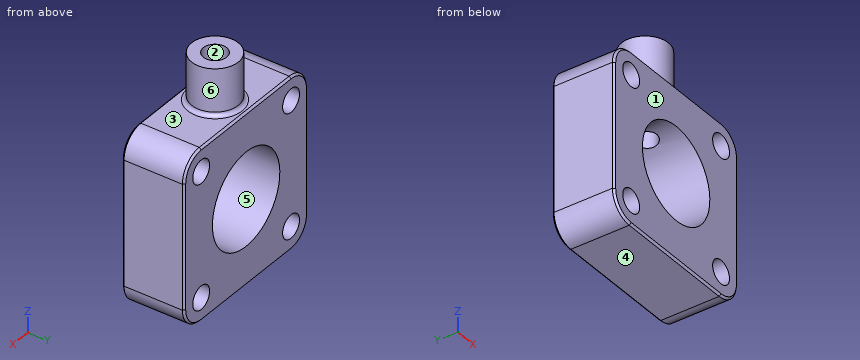
```python
from build123d import *

# Parameters (mm, degrees)
SKETCH1_R           = 1.5
SKETCH1_R_2         = 6
BOSS_EXTRUDE1_DEPTH = 4
BOSS_EXTRUDE2_START = 11
SKETCH2_R           = 3
BOSS_EXTRUDE2_DEPTH = 6
SKETCH3_R           = 1.5
CUT_EXTRUDE1_DEPTH  = 16
CHAMFER1_SIZE       = 0.25
FILLET1_R           = 0.5


with BuildPart() as part:
    # Sketch1 → Boss-Extrude1 (new, symmetric)
    with BuildSketch(Plane(origin=(0, 0, 0), x_dir=(1, 0, 0), z_dir=(0, 1, 0))):
        with BuildLine():
            Line((8, -11), (-8, -11))
            ThreePointArc((-8, -11), (-10.121320344, -10.121320344), (-11, -8))
            Line((-11, -8), (-11, 8))
            ThreePointArc((-11, 8), (-10.121320344, 10.121320344), (-8, 11))
            Line((-8, 11), (8, 11))
            ThreePointArc((8, 11), (10.121320344, 10.121320344), (11, 8))
            Line((11, 8), (11, -8))
            ThreePointArc((11, -8), (10.121320344, -10.121320344), (8, -11))
        make_face()
        with Locations(Location((-8, 8, 0), (0, 0, 270))):
            Circle(SKETCH1_R, mode=Mode.SUBTRACT)
        with Locations(Location((8, 8, 0), (0, 0, 270))):
            Circle(SKETCH1_R, mode=Mode.SUBTRACT)
        with Locations(Location((8, -8, 0), (0, 0, 270))):
            Circle(SKETCH1_R, mode=Mode.SUBTRACT)
        with Locations(Location((-8, -8, 0), (0, 0, 270))):
            Circle(SKETCH1_R, mode=Mode.SUBTRACT)
        with Locations(Location((0, 0, 0), (0, 0, 270))):
            Circle(SKETCH1_R_2, mode=Mode.SUBTRACT)
    extrude(amount=BOSS_EXTRUDE1_DEPTH, both=True)

    # Sketch2 → Boss-Extrude2 (add)
    with BuildSketch(Plane.XY.offset(BOSS_EXTRUDE2_START)):
        with Locations(Location((0, 0, 0), (0, 0, 180))):
            Circle(SKETCH2_R)
    extrude(amount=BOSS_EXTRUDE2_DEPTH)

    # Sketch3 → Cut-Extrude1 (cut)
    with BuildSketch(Plane.XY.offset(17)):
        Circle(SKETCH3_R)
    extrude(amount=-CUT_EXTRUDE1_DEPTH, mode=Mode.SUBTRACT)

    # Chamfer1
    chamfer1_edges = [part.edges().sort_by_distance(p)[0] for p in [
        (0, -4, -11),
        (10.121320344, -4, -10.121320344),
        (11, -4, 0),
        (10.121320344, -4, 10.121320344),
        (10.121320344, 4, -10.121320344),
        (0, 4, -11),
        (-10.121320344, 4, -10.121320344),
        (-11, 4, 0),
        (-10.121320344, 4, 10.121320344),
        (0, 4, 11),
        (10.121320344, 4, 10.121320344),
        (0, -4, 11),
        (11, 4, 0),
        (-10.121320344, -4, 10.121320344),
        (-11, -4, 0),
        (-10.121320344, -4, -10.121320344),
    ]]
    chamfer(chamfer1_edges, length=CHAMFER1_SIZE)

    # Fillet1
    fillet1_edges = [part.edges().sort_by_distance(p)[0] for p in [
        (3, 0, 11),
    ]]
    fillet(fillet1_edges, radius=FILLET1_R)


solid = part.part
```
Verification items for the finished model (mm, model axes). Face numbers are marked on the shaded views. A direction names the side the tool comes from. Round coordinates to 2 decimals unless told otherwise and drop trailing zeros. Order: outer loops, then holes, each group sorted by start corner. A loop starts at its lowest first (then second) coordinate and runs counter-clockwise, first axis right, second up.
1) Depth check by flat-ended pin: pin 1 (2.5 mm diameter, centred on x = 0, y = 0, fed in from +Z). Enter the tip coordinate at first touch or a pass-through.
Geometry says:
pin 1: stops at z = -5.87
2) Cross-section at A-A, the plane x = 0. Record the cut outline in (y, z).
Geometry says:
outline: (-4, -10.75) - (-3.75, -11) - (3.75, -11) - (4, -10.75) - (4, -6) - (-4, -6) - close; (-4, 6) - (-1.5, 6) - (-1.5, 17) - (-3, 17) - (-3, 11.5) arc R0.5 cw to (-3.5, 11) - (-3.75, 11) - (-4, 10.75) - close; (1.5, 6) - (4, 6) - (4, 10.75) - (3.75, 11) - (3.5, 11) arc R0.5 cw to (3, 11.5) - (3, 17) - (1.5, 17) - close
3) Draft check along Z on the marked faces 3, 4, 5 and 6. Enter one of: +Z half, -Z half, draft (parallel to the pull), parting line (faces both ways), or undercut.
Geometry says:
face 3: +Z half
face 4: -Z half
face 5: undercut
face 6: draft
4) Cross-section at C-C, the plane x = -4. Record the cut outline in (y, z), plus the area to 3 significant figures.
Geometry says:
outline: (-4, -10.75) - (-3.75, -11) - (3.75, -11) - (4, -10.75) - (4, -4.47) - (-4, -4.47) - close; (-4, 4.47) - (4, 4.47) - (4, 10.75) - (3.75, 11) - (-3.75, 11) - (-4, 10.75) - close
area: 104 mm2
5) Cross-section at B-B, the plane y = 0. Record the cut outline in (x, z).
Geometry says:
outline: (-11, -8) arc R3 ccw to (-8, -11) - (8, -11) arc R3 ccw to (11, -8) - (11, 8) arc R3 ccw to (8, 11) - (3.5, 11) arc R0.5 cw to (3, 11.5) - (3, 17) - (1.5, 17) - (1.5, 5.81) arc R6 cw (long way) to (-1.5, 5.81) - (-1.5, 17) - (-3, 17) - (-3, 11.5) arc R0.5 cw to (-3.5, 11) - (-8, 11) arc R3 ccw to (-11, 8) - close; hole circle Ø3 at (-8, -8); hole circle Ø3 at (-8, 8); hole circle Ø3 at (8, -8); hole circle Ø3 at (8, 8)
6) Tool access check on the marked faces 1 and 2. Record the directions out of +Z, -Z, +X, -X, +Y, -Y that give a thin tool (end or side, any length) a straight path to the whole face; none if there is none.
Geometry says:
face 1: +Z, -Z, +X, -X, -Y
face 2: +Z
7) Cross-section at D-D, the plane z = 3.5. Record the cut outline in (x, y).
Geometry says:
outline: (-11, -3.75) - (-10.75, -4) - (-4.87, -4) - (-4.87, 4) - (-10.75, 4) - (-11, 3.75) - close; (4.87, -4) - (10.75, -4) - (11, -3.75) - (11, 3.75) - (10.75, 4) - (4.87, 4) - close
8) Material ranges on line 1 (X direction, y = -2, z = -8); line 2 (Y direction, x = 0, z = 14.75); line 3 (X direction, y = -1, z = 0), recorded low to high.
Geometry says:
line 1: x = -11 to -9.5, -6.5 to 6.5, 9.5 to 11
line 2: y = -3 to -1.5, 1.5 to 3
line 3: x = -11 to -6, 6 to 11
